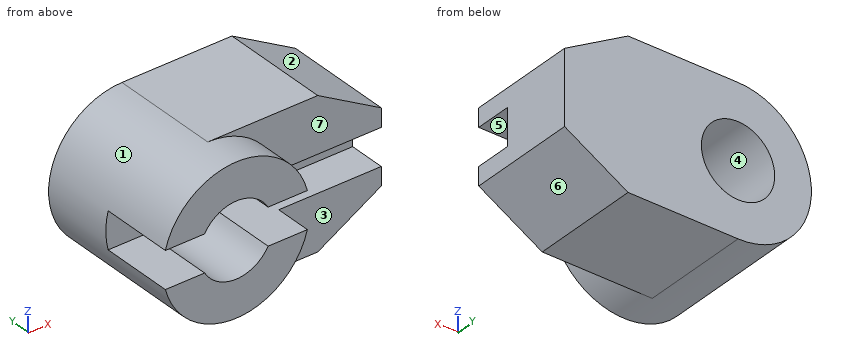
```python
from build123d import *

# Parameters (mm, degrees)
F0_R     = 10
F0_R_2   = 5
F1_DEPTH = 20
F3_START = -5
F3_DEPTH = 15
F4_W     = 5
F4_H     = 5
F5_DEPTH = 33.6612540378


with BuildPart() as f1:
    # F0 (on Front) → F1 (new body)
    with BuildSketch(Plane.XZ):
        Circle(F0_R)
        Circle(F0_R_2, mode=Mode.SUBTRACT)
    extrude(amount=F1_DEPTH)

    # F2 (on face) → F3 (join)
    with BuildSketch(Plane.XZ.offset(20).offset(F3_START)):
        Polygon((23.6602540378, 5), (15, 10), (15, -10), (23.6602540378, -5), align=None)
        with BuildLine():
            Line((15, 10), (0, 10))
            ThreePointArc((0, 10), (7.0710678119, 7.0710678119), (10, 0))
            ThreePointArc((10, 0), (7.0710678119, -7.0710678119), (0, -10))
            Line((0, -10), (15, -10))
            Line((15, -10), (15, 10))
        make_face()
    extrude(amount=-F3_DEPTH)

    # F4 (on face) → F5 (cut, through all)
    with BuildSketch(Plane.YZ.offset(23.6602540378)):
        with Locations((-12.5, 0)):
            Rectangle(F4_W, F4_H)
        with Locations((-17.5, 0)):
            Rectangle(F4_W, F4_H)
    extrude(amount=-F5_DEPTH, mode=Mode.SUBTRACT)


solid = f1.part
```
Verification items for the finished model (mm, model axes). Face numbers are marked on the shaded views. A direction names the side the tool comes from. Coordinates: 2 decimals unless noted, no trailing zeros. Loops run counter-clockwise (first coordinate to the right, second up) from the corner with the lowest first, then second, coordinate; pieces in that order, holes last. Notation, with made-up numbers: (88, -7.75) - (103, -7.75) arc R30 cw to (103, 30.25) - close; hole circle Ø11 at (60, -16.75). An arc over 180 degrees is marked (long way). Return JSON: item names as keys, results as strings.
1. Section check A-A, the plane y = -16. Record the boundary of the cut face in (x, z), then the cut area to 3 significant figures.
Established:
{"outline": "(-9.68, -2.5) arc R10 ccw to (9.68, -2.5) - (4.33, -2.5) arc R5 cw to (-4.33, -2.5) - close; (-9.68, 2.5) - (-4.33, 2.5) arc R5 cw to (4.33, 2.5) - (9.68, 2.5) arc R10 ccw to start", "area": "185 mm2"}
2. Go/stop test with flat-tipped pins: pin 1 (4.5 mm diameter, centred on x = -6, y = -13, fed in from +Z); pin 2 (4 mm diameter, centred on x = 15, z = -1, fed in from -Y); pin 3 (1 mm diameter, centred on y = -2.5, z = 7.5, fed in from -X); pin 4 (3 mm diameter, centred on x = 18, y = -17.5, fed in from -Z). Record where each tip stops, or that it passes through.
Established:
{"pin 1": "stops at z = 9.27", "pin 2": "stops at y = -15", "pin 3": "stops at x = -7.14", "pin 4": "passes through"}
3. Section check C-C, the plane z = 0. Record the boundary of the cut face in (x, y).
Established:
{"outline": "(-10, -10) - (-5, -10) - (-5, 0) - (-10, 0) - close; (5, -10) - (23.66, -10) - (23.66, 0) - (5, 0) - close"}
4. Mould release check, pull along X, two halves, no side actions. Record for the marked faces 1, 2, 3 and 4: +X half, -X half, draft (parallel to the pull), parting line (faces both ways), or undercut.
Established:
{"face 1": "parting line", "face 2": "+X half", "face 3": "draft", "face 4": "undercut"}
5. Section check B-B, the plane x = 2.5. Record the boundary of the cut face in (y, z).
Established:
{"outline": "(-20, -9.68) - (-15, -9.68) - (-15, -10) - (0, -10) - (0, -4.33) - (-20, -4.33) - close; (-20, 4.33) - (0, 4.33) - (0, 10) - (-15, 10) - (-15, 9.68) - (-20, 9.68) - close"}
6. Tool access check on the marked faces 5, 6 and 7. Record the directions out of +Z, -Z, +X, -X, +Y, -Y that give a thin tool (end or side, any length) a straight path to the whole face; none if there is none.
Established:
{"face 5": "+X, -X, -Y", "face 6": "-Z, +X, +Y, -Y", "face 7": "+Z, +X, -Y"}
7. Section check D-D, the plane y = -8.75. Record the boundary of the cut face in (x, z), then the cut area to 3 significant figures.
Established:
{"outline": "(0, -10) - (15, -10) - (23.66, -5) - (23.66, 5) - (15, 10) - (0, 10) arc R10 ccw to start; hole circle Ø10 at (0, 0)", "area": "508 mm2"}
8. Thickness scan on L1, parallel to X at y = -9, z = 0; L2, parallel to Z at x = 0, y = -4.75; L3, parallel to Z at x = 4, y = -12.25. Record the ranges inside material, lowest first.
Established:
{"L1": "x = -10 to -5, 5 to 23.66", "L2": "z = -10 to -5, 5 to 10", "L3": "z = -10 to -3, 3 to 10"}
